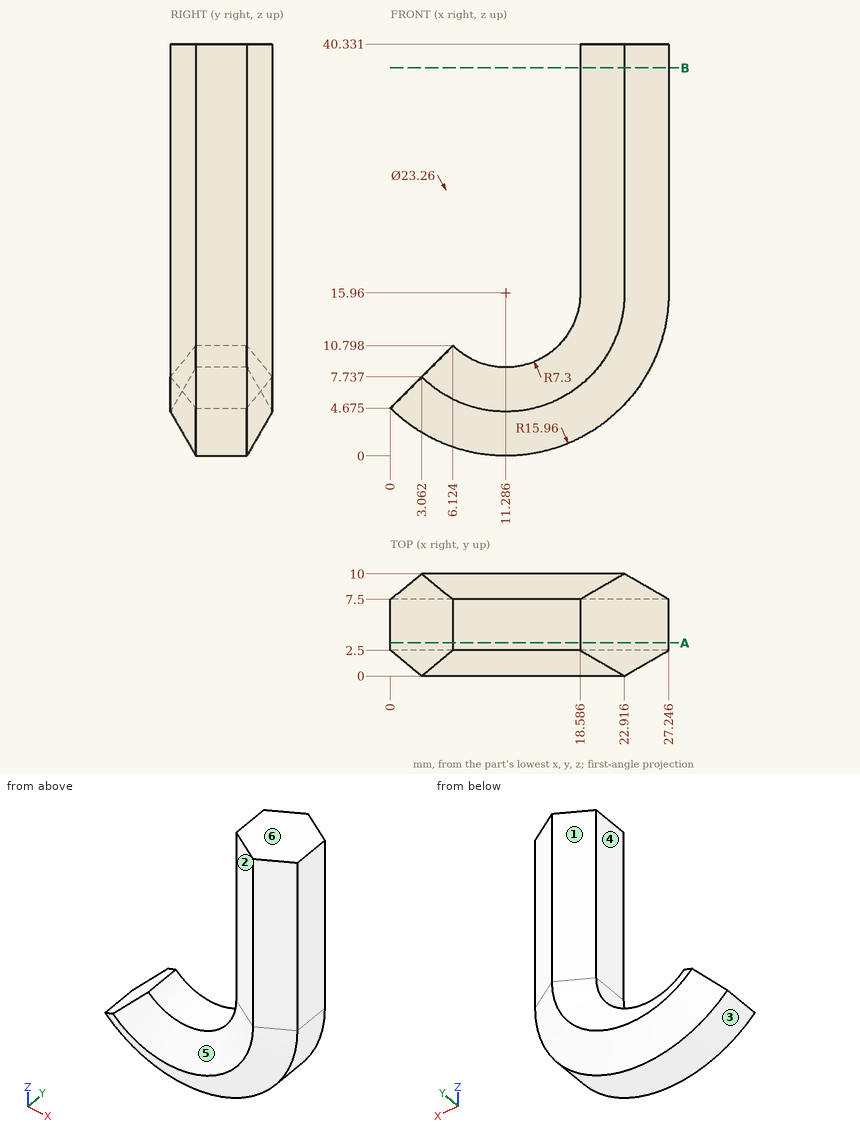
Check sheet for the drawn part. Datum: minimum x, y, z corner. Units: mm. A direction names the side the tool comes from. Round coordinates to 2 decimals unless told otherwise and drop trailing zeros. Order: outer loops, then holes, each group sorted by start corner. A loop starts at its lowest first (then second) coordinate and runs counter-clockwise, first axis right, second up. Notation, with made-up numbers: (38, 84) - (94, 84) arc R10 ccw to (94, 95) - close; hole circle Ø4 at (-14.5, 20.5). An arc over 180 degrees is marked (long way). Use a Markdown table: item, result. Add a question column.
(1) Sectioned sample at B-B, the plane z = 38. Enter the section's corners in (x, y) (1 decimal).
(2) Tool access check on the marked faces 1, 2 and 3. Record the directions out of +Z, -Z, +X, -X, +Y, -Y that give a thin tool (end or side, any length) a straight path to the whole face; none if there is none.
(3) Depth check by flat-ended pin: pin 1 (1.5 mm diameter, centred on x = 18.5, z = 33, fed in from -Y) (1 decimal); pin 2 (4 mm diameter, centred on y = 4.5, z = 25.5, fed in from -X); pin 3 (1.5 mm diameter, centred on x = 15.5, y = 8, fed in from -Z) (1 decimal). Enter the tip coordinate at first touch or a pass-through.
(4) Material ranges on line 1 along X through (y, z) = (6, 20) (1 decimal); line 2 along X through (y, z) = (5, 12.5) (1 decimal); line 3 along Z through (x, y) = (22.25, 7) (1 decimal), recorded low to high. Write a range as [from, to].
(5) Release check for a two-part mould opening along X. For the marked faces 4, 5 and 6 record: pulls with the +X half, pulls with the -X half, needs draft (parallel to the pull), parting line crosses it, or undercut.
(6) Sectioned sample at A-A, the plane y = 3.25. Enter the section's corners in (x, z) (1 decimal).
Answers below:
| question | item | result |
|---|---|---|
| 1 | outline | (18.6, 2.5) - (22.9, 0) - (27.2, 2.5) - (27.2, 7.5) - (22.9, 10) - (18.6, 7.5) - close |
| 2 | face 1 | +Z, -X, +Y |
| 2 | face 2 | +Z, -X, -Y |
| 2 | face 3 | -Z, +Y, -Y |
| 3 | pin 1 | y = 2.1 |
| 3 | pin 2 | x = 18.59 |
| 3 | pin 3 | z = 0.4 |
| 4 | line 1 | [18.6, 27.2] |
| 4 | line 2 | [17.7, 26.9] |
| 4 | line 3 | [4.4, 40.3] |
| 5 | face 4 | pulls with the -X half |
| 5 | face 5 | undercut |
| 5 | face 6 | needs draft |
| 6 | outline | (0, 4.7) arc R16 ccw to (27.2, 16) - (27.2, 40.3) - (18.6, 40.3) - (18.6, 16) arc R7.3 cw to (6.1, 10.8) - close |
